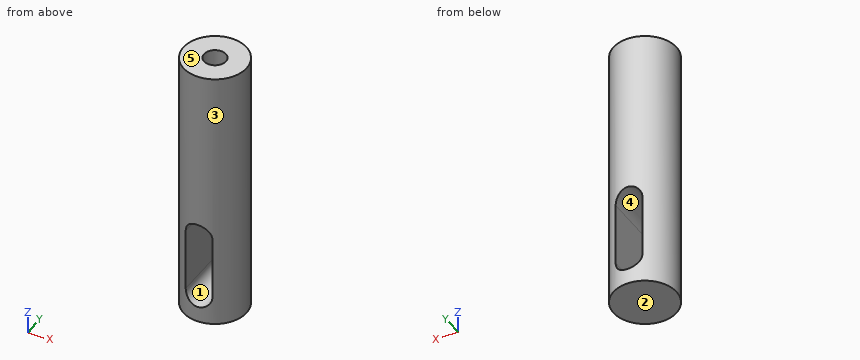
```python
from build123d import *

# Parameters (mm, degrees)
F0_R          = 5.08
F0_R_2        = 1.778
F1_DEPTH      = 25.4
F2_DEPTH      = 43.18
F4_DEPTH      = 25.4
F4_DEPTH_BACK = 25.4


with BuildPart() as f1:
    # F0 (on Top) → F1 (new body)
    with BuildSketch(Plane.XY):
        Circle(F0_R)
        Circle(F0_R_2, mode=Mode.SUBTRACT)
        Circle(F0_R_2)
    extrude(amount=F1_DEPTH)

    # F0 (on Top) → F2 (join)
    with BuildSketch(Plane.XY):
        Circle(F0_R)
        Circle(F0_R_2, mode=Mode.SUBTRACT)
    extrude(amount=F2_DEPTH)

    # F3 (on Front) → F4 (cut, two sides)
    with BuildSketch(Plane.XZ) as f4_sk:
        with BuildLine():
            ThreePointArc((-2.159, 4.699), (0, 2.54), (2.159, 4.699))
            ThreePointArc((2.159, 4.699), (0, 6.858), (-2.159, 4.699))
        make_face()
        with BuildLine():
            ThreePointArc((-2.159, 4.699), (0, 6.858), (2.159, 4.699))
            Line((2.159, 4.699), (2.159, 14.859))
            ThreePointArc((2.159, 14.859), (0, 12.7), (-2.159, 14.859))
            Line((-2.159, 14.859), (-2.159, 4.699))
        make_face()
        with BuildLine():
            ThreePointArc((-2.159, 14.859), (0, 12.7), (2.159, 14.859))
            ThreePointArc((2.159, 14.859), (0, 17.018), (-2.159, 14.859))
        make_face()
    extrude(amount=-F4_DEPTH, mode=Mode.SUBTRACT)
    extrude(f4_sk.sketch, amount=F4_DEPTH_BACK, mode=Mode.SUBTRACT)


solid = f1.part
```
Design review of the part built by this model. Coordinates are the model's own, in mm. Face numbers are marked on the shaded views. A direction names the side the tool comes from. Round coordinates to 2 decimals unless told otherwise and drop trailing zeros. Order: outer loops, then holes, each group sorted by start corner. A loop starts at its lowest first (then second) coordinate and runs counter-clockwise, first axis right, second up. Notation, with made-up numbers: M 0.5,-34 L 41.5,-34 A18 cw 41.5,-16 Z; hole C 2,6 d3. An arc over 180 degrees is marked long. Put each result on its own line as item: value.
Q1. Consider section A-A (y = 0). State the section outline as (x, z) points.
Reported:
outline: M -5.08,0 L 5.08,0 L 5.08,43.18 L 1.78,43.18 L 1.78,25.4 L -1.78,25.4 L -1.78,43.18 L -5.08,43.18 Z; hole M -2.16,4.7 A2.16 ccw 2.16,4.7 L 2.16,14.86 A2.16 ccw -2.16,14.86 Z
Q2. Consider section B-B (x = 0). State the section outline as (y, z) points, and give its area (3 significant figures).
Reported:
outline: M -5.08,0 L 5.08,0 L 5.08,2.54 L -5.08,2.54 Z; M -5.08,17.02 L 5.08,17.02 L 5.08,43.18 L 1.78,43.18 L 1.78,25.4 L -1.78,25.4 L -1.78,43.18 L -5.08,43.18 Z
area: 228 mm²
Q3. To check wall thickness, follow line 1 (Y direction, x = 0, z = 38.5); line 2 (Z direction, x = 0, y = 0.75); line 3 (X direction, y = -2.25, z = 15). State the ranges of each line that lie inside material, in increasing order.
Reported:
line 1: -5.08 to -1.78, 1.78 to 5.08
line 2: 0 to 2.54, 17.02 to 25.4
line 3: -4.55 to -2.15, 2.15 to 4.55
Q4. Consider section D-D (y = -3). State the section outline as (x, z) points, and give its area (3 significant figures).
Reported:
outline: M -4.1,0 L 4.1,0 L 4.1,43.18 L -4.1,43.18 Z; hole M -2.16,4.7 A2.16 ccw 2.16,4.7 L 2.16,14.86 A2.16 ccw -2.16,14.86 Z
area: 296 mm²
Q5. Draft analysis for pull direction X (two halves, no side actions). For the marked faces 3, 4 and 5, state which applies: released by +X, released by -X, zero draft, split by the parting line, or undercut.
Reported:
face 3: split by the parting line
face 4: undercut
face 5: zero draft
Q6. Insertion check: pin 1 Ø3 at (y, z) = (-2, 12) entering from +X; pin 2 Ø1.1 at (x, y) = (0, -1) entering from +Z; pin 3 Ø1.5 at (y, z) = (3.5, 21) entering from +X. Each pin has a flat end and moves straight along its axis. Give the tip position at first contact, or say it passes through.
Reported:
pin 1: x = 5.06
pin 2: z = 25.4
pin 3: x = 4.27
Q7. Machinability: for the marked faces 1 and 2, which of the approach directions +Z, -Z, +X, -X, +Y, -Y give a long, thin tool a straight path to every point of the face, cutting with its end or side? Answer none if there is none.
Reported:
face 1: +Y, -Y
face 2: -Z, +X, -X, +Y, -Y
Q8. Consider section C-C (z = 38.5). State the section outline as (x, y) points.
Reported:
outline: C 0,0 d10.16; hole C 0,0 d3.56
